Input: part model. Units: mm. Frame: model coordinates. A direction names the side the tool comes from. Coordinates: 2 decimals unless noted, no trailing zeros. Order: outer loops, then holes, each group sorted by start corner. A loop starts at its lowest first (then second) coordinate and runs counter-clockwise, first axis right, second up. Notation, with made-up numbers: (86, -24.5) -> (124, -24.5) arc R20 cw to (124, 9.5) -> close; hole circle Ø10 at (81.25, -33). An arc over 180 degrees is marked (long way). One line per question, with ' | ' between items.
```python
from build123d import *

# Parameters (mm, degrees)
SKETCH004_R  = 4
PAD004_DEPTH = 10
SKETCH001_W  = 28
SKETCH001_H  = 19
PAD001_DEPTH = 2
PAD002_DEPTH = 1
SKETCH003_R  = 8
PAD003_DEPTH = 5
SKETCH_W     = 28
SKETCH_H     = 19
PAD_DEPTH    = 2
FILLET_R     = 1.5


with BuildPart() as body004:
    # Sketch004 → Pad004 (new body)
    with BuildSketch(Plane.XY):
        Circle(SKETCH004_R)
    extrude(amount=PAD004_DEPTH)


with BuildPart() as body001:
    # Sketch001 → Pad001 (new body)
    with BuildSketch(Plane.XY):
        Rectangle(SKETCH001_W, SKETCH001_H)
    extrude(amount=PAD001_DEPTH)


with BuildPart() as body001_1:
    # Body001 placement: moved
    add(body001.part.moved(Location((0, 0, 3))))


with BuildPart() as body002:
    # Sketch002 → Pad002 (new body)
    with BuildSketch(Plane.XY):
        with BuildLine():
            ThreePointArc((-10, 3), (0, -7), (10, 3))
            Line((10, 9.5), (10, 3))
            Line((-10, 9.5), (10, 9.5))
            Line((-10, 3), (-10, 9.5))
        make_face()
    extrude(amount=PAD002_DEPTH)


with BuildPart() as body002_1:
    # Body002 placement: moved
    add(body002.part.moved(Location((0, 0, 2))))


with BuildPart() as body003:
    # Sketch003 → Pad003 (new body)
    with BuildSketch(Plane.XY):
        Circle(SKETCH003_R)
    extrude(amount=PAD003_DEPTH)


with BuildPart() as body003_1:
    # Body003 placement: moved
    add(body003.part.moved(Location((0, 0, 5))))


with BuildPart() as fillet_body:
    # Sketch → Pad (new body)
    with BuildSketch(Plane.XY):
        Rectangle(SKETCH_W, SKETCH_H)
    extrude(amount=PAD_DEPTH)

    # Fusion: union Body001, Body002, Body003
    add(body001_1.part)
    add(body002_1.part)
    add(body003_1.part)

    # Cut: cut Body004
    add(body004.part, mode=Mode.SUBTRACT)

    # Fillet
    fillet_edges = [fillet_body.edges().sort_by_distance(p)[0] for p in [
        (-8, 0, 10),
    ]]
    fillet(fillet_edges, radius=FILLET_R)


solid = fillet_body.part
```
1. Cut plane B-B, the plane z = 2.5. Return loops of the section in (x, y), and give its area (3 significant figures).
Recorded:
outline: (-10, 3) arc R10 ccw to (10, 3) -> (10, 9.5) -> (-10, 9.5) -> close; hole circle Ø8 at (0, 0) | area: 237 mm^2
2. Cut plane D-D, the plane x = 11.25. Return loops of the section in (y, z).
Recorded:
outline: (-9.5, 0) -> (9.5, 0) -> (9.5, 2) -> (-9.5, 2) -> close; (-9.5, 3) -> (9.5, 3) -> (9.5, 5) -> (-9.5, 5) -> close
3. Mould query, pull axis Z, two halves, no side actions, for faces 5 (the face through (-0.2, -8.3, 5)), 6 (the face through (0, -8, 3)), 7 (the face through (-0.2, 4.4, 0)), 8 (the face through (-14, 0, 1)). Classes: released by +Z, released by -Z, zero draft, split by the parting line, or undercut.
Recorded:
face 5: released by +Z | face 6: undercut | face 7: released by -Z | face 8: zero draft
4. Cut plane A-A, the plane x = 0. Return loops of the section in (y, z), and give its area (3 significant figures).
Recorded:
outline: (-9.5, 0) -> (-4, 0) -> (-4, 10) -> (-6.5, 10) arc R1.5 ccw to (-8, 8.5) -> (-8, 5) -> (-9.5, 5) -> (-9.5, 3) -> (-7, 3) -> (-7, 2) -> (-9.5, 2) -> close; (4, 0) -> (9.5, 0) -> (9.5, 5) -> (8, 5) -> (8, 8.5) arc R1.5 ccw to (6.5, 10) -> (4, 10) -> close | area: 91.5 mm^2
5. Pin query (flat end, axial travel): pin 1 Ø1 at (x, y) = (3.5, 3) entering from -Z; pin 2 Ø5 at (x, y) = (0, 0) entering from -Z; pin 3 Ø1.5 at (x, y) = (-8, 3) entering from +Z; pin 4 Ø0.8 at (y, z) = (5.5, 2.5) entering from -X. Return the tip coordinate at first contact, or that it passes through.
Recorded:
pin 1: stops at z = 0 | pin 2: passes through | pin 3: stops at z = 9.26 | pin 4: stops at x = -10
6. Ray query, line 1 (Z direction, x = -8, y = -6.5); line 2 (Y direction, x = 0, z = 3.25); line 3 (Y direction, x = 2.25, z = 4.5). Return the intervals inside material, ascending. Write a range as [from, to].
Recorded:
line 1: z = [0, 2], [3, 5] | line 2: y = [-9.5, -4], [4, 9.5] | line 3: y = [-9.5, -3.31], [3.31, 9.5]
7. Cut plane C-C, the plane y = 0. Return loops of the section in (x, z), and give its area (3 significant figures).
Recorded:
outline: (-14, 0) -> (-4, 0) -> (-4, 10) -> (-6.5, 10) arc R1.5 ccw to (-8, 8.5) -> (-8, 5) -> (-14, 5) -> (-14, 3) -> (-9.54, 3) -> (-9.54, 2) -> (-14, 2) -> close; (4, 0) -> (14, 0) -> (14, 2) -> (9.54, 2) -> (9.54, 3) -> (14, 3) -> (14, 5) -> (8, 5) -> (8, 8.5) arc R1.5 ccw to (6.5, 10) -> (4, 10) -> close | area: 130 mm^2
8. Access query for faces 1 (the face through (-1.73, -7.81, 6.73)), 2 (the face through (10, 6.3, 2.5)), 3 (the face through (-10, 6.2, 2.5)), 4 (the face through (-0.2, -7, 2.5)). Directions: +Z, -Z, +X, -X, +Y, -Y. A direction counts if a zero-diameter tool reaches every point of the face in a straight line with its end or side. Return the directions, or none.
Recorded:
face 1: +Z | face 2: +X, +Y, -Y | face 3: -X, +Y, -Y | face 4: -Y
